Part model, mm, in its own coordinate system. Face numbers are marked on the shaded views. A direction names the side the tool comes from. Round coordinates to 2 decimals unless told otherwise and drop trailing zeros. Order: outer loops, then holes, each group sorted by start corner. A loop starts at its lowest first (then second) coordinate and runs counter-clockwise, first axis right, second up. Notation, with made-up numbers: (28.5, 34.25) -> (58.5, 34.25) arc R33 cw to (58.5, 69.25) -> close; hole circle Ø5 at (23.25, 42.25). An arc over 180 degrees is marked (long way). Use CSV: the item, a comma, the result in double quotes.
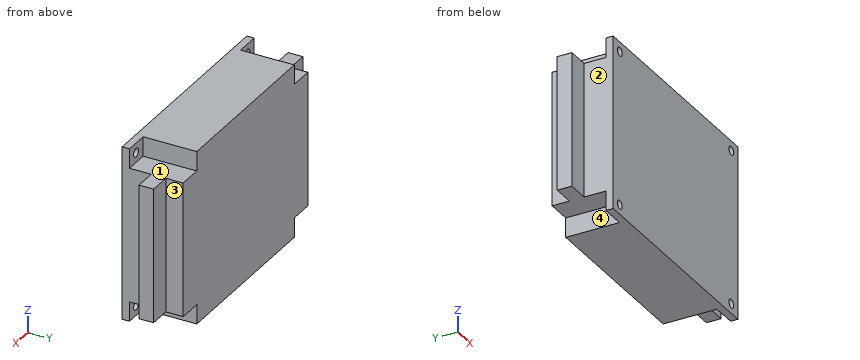
```python
from build123d import *

# Parameters (mm, degrees)
SKETCH_1_W             = 91.7
SKETCH_1_H             = 71
EXTRUDE_1_DEPTH        = 25
SKETCH_2_W             = 10.00292335
SKETCH_2_H             = 22
CUT_EXTRUDE_1_DEPTH    = 8.000270383
SKETCH_3_W             = 54.999459234
SKETCH_3_H             = 13.1
EXTRUDE_2_DEPTH        = 9
SKETCH_4_W             = 8.000270383
SKETCH_4_H             = 22
CUT_EXTRUDE_2_DEPTH    = 10.00292335
SKETCH_5_W             = 8.000270383
SKETCH_5_H             = 22
CUT_EXTRUDE_3_DEPTH    = 10.00292335
SKETCH_6_W             = 54.999459234
SKETCH_6_H             = 13.1
EXTRUDE_3_DEPTH        = 9
SKETCH_7_W             = 8.000270383
SKETCH_7_H             = 22
CUT_EXTRUDE_4_DEPTH    = 10.00292335
SKETCH_8_W             = 9
SKETCH_8_H             = 7.1
CUT_EXTRUDE_5_DEPTH    = 122.38556723
SKETCH_9_W             = 9
SKETCH_9_H             = 7.1
CUT_EXTRUDE_6_DEPTH    = 122.38556723
HOLE_WIZARD_M3_1_D     = 3.531196766
HOLE_WIZARD_M3_1_DEPTH = 25


with BuildPart() as part:
    # 草图1 → 凸台-拉伸1 (new body)
    with BuildSketch(Plane(origin=(0, 25, 0), x_dir=(1, 0, 0), z_dir=(0, 1, 0))):
        with Locations((45.85, 24.5)):
            Rectangle(SKETCH_1_W, SKETCH_1_H)
    extrude(amount=-EXTRUDE_1_DEPTH)

    # 草图2 → 切除-拉伸1 (cut)
    with BuildSketch(Plane(origin=(0, 0, -60), x_dir=(-1, 0, 0), z_dir=(0, 0, -1))):
        with Locations((-5.001461675, 14)):
            Rectangle(SKETCH_2_W, SKETCH_2_H)
    extrude(amount=-CUT_EXTRUDE_1_DEPTH, mode=Mode.SUBTRACT)

    # 草图3 → 凸台-拉伸2 (add)
    with BuildSketch(Plane.ZY):
        with Locations((-24.5, 18.45)):
            Rectangle(SKETCH_3_W, SKETCH_3_H)
    extrude(amount=EXTRUDE_2_DEPTH)

    # 草图4 → 切除-拉伸2 (cut)
    with BuildSketch(Plane.ZY):
        with Locations((6.999864808, 14)):
            Rectangle(SKETCH_4_W, SKETCH_4_H)
    extrude(amount=-CUT_EXTRUDE_2_DEPTH, mode=Mode.SUBTRACT)

    # 草图5 → 切除-拉伸3 (cut)
    with BuildSketch(Plane(origin=(91.7, 0, 0), x_dir=(0, 0, -1), z_dir=(1, 0, 0))):
        with Locations((55.999864809, 14)):
            Rectangle(SKETCH_5_W, SKETCH_5_H)
    extrude(amount=-CUT_EXTRUDE_3_DEPTH, mode=Mode.SUBTRACT)

    # 草图6 → 凸台-拉伸3 (add)
    with BuildSketch(Plane(origin=(91.7, 0, 0), x_dir=(0, 0, -1), z_dir=(1, 0, 0))):
        with Locations((24.5, 18.45)):
            Rectangle(SKETCH_6_W, SKETCH_6_H)
    extrude(amount=EXTRUDE_3_DEPTH)

    # 草图7 → 切除-拉伸4 (cut)
    with BuildSketch(Plane(origin=(91.7, 0, 0), x_dir=(0, 0, -1), z_dir=(1, 0, 0))):
        with Locations((-6.999864808, 14)):
            Rectangle(SKETCH_7_W, SKETCH_7_H)
    extrude(amount=-CUT_EXTRUDE_4_DEPTH, mode=Mode.SUBTRACT)

    # 草图8 → 切除-拉伸5 (cut, through all)
    with BuildSketch(Plane(origin=(0, 0, -51.999729617), x_dir=(-1, 0, 0), z_dir=(0, 0, -1))):
        with Locations((4.5, 21.45)):
            Rectangle(SKETCH_8_W, SKETCH_8_H)
    extrude(amount=-CUT_EXTRUDE_5_DEPTH, mode=Mode.SUBTRACT)

    # 草图9 → 切除-拉伸6 (cut, through all)
    with BuildSketch(Plane.XY.offset(2.999729617)):
        with Locations((96.2, 21.45)):
            Rectangle(SKETCH_9_W, SKETCH_9_H)
    extrude(amount=-CUT_EXTRUDE_6_DEPTH, mode=Mode.SUBTRACT)

    # M3 间隙孔1
    with Locations(Plane(origin=(0, 0, 0), x_dir=(-1, 0, 0), z_dir=(0, -1, 0))):
        with Locations((-86.846324066, 55.999601401), (-86.846324066, -6.999601401), (-4.853675934, -6.999601401), (-4.853675934, 55.999601401)):
            Hole(HOLE_WIZARD_M3_1_D / 2, depth=HOLE_WIZARD_M3_1_DEPTH)


solid = part.part
```
(1) Which spindle directions (+Z, -Z, +X, -X, +Y, -Y) get a long thin tool onto all of the face, cutting with end or side? Do the marked faces 1, 2, 3 and 4. Say none if no direction does.
Reply:
face 1,"+Z, +X, +Y"
face 2,"+Z, -Z, -X, -Y"
face 3,"+Z, -Z, +X, +Y"
face 4,"-Z, -X, +Y"
(2) Probe probe 1 along X at (y, z) = (21, -35.5); probe 2 along X at (y, z) = (14.5, -53.5); probe 3 along Z at (x, y) = (88, 11). List the from-to ranges inside material, lowest first. Write a range as [from, to].
Reply:
probe 1,"[0, 91.7]"
probe 2,"[10, 81.7]"
probe 3,"[-52, 3]"
(3) Cut at A-A, the plane y = 16.25. Give the cut face in (x, z), then the cut area to 3 significant figures.
Reply:
outline,"(-9, -52) -> (10, -52) -> (10, -60) -> (81.7, -60) -> (81.7, -52) -> (100.7, -52) -> (100.7, 3) -> (81.7, 3) -> (81.7, 11) -> (10, 11) -> (10, 3) -> (-9, 3) -> close"
area,"7,180 mm2"
(4) Cut at B-B, the plane z = -11. Give the cut face in (x, y), then the cut area to 3 significant figures.
Reply:
outline,"(-9, 11.9) -> (0, 11.9) -> (0, 0) -> (91.7, 0) -> (91.7, 11.9) -> (100.7, 11.9) -> (100.7, 17.9) -> (91.7, 17.9) -> (91.7, 25) -> (0, 25) -> (0, 17.9) -> (-9, 17.9) -> close"
area,"2,400 mm2"
(5) Drop flat-ended pins along their axis: P1, Ø5.5, axis at x = 3, y = 17, coming from the -Z side; P2, Ø6, axis at y = 5.5, z = -13, coming from the -X side; P3, Ø2.5, axis at x = 4, z = -55.5, coming from the +Y side. Give the stop position or say it passes through.
Reply:
P1,"z = -52"
P2,"x = 0"
P3,"y = 3"
(6) Cut at C-C, the plane x = 87. Give the cut face in (y, z), then the cut area to 3 significant figures.
Reply:
outline,"(0, -60) -> (3, -60) -> (3, -57.76) -> (0, -57.76) -> close; (0, -54.24) -> (3, -54.24) -> (3, -52) -> (25, -52) -> (25, 3) -> (3, 3) -> (3, 5.24) -> (0, 5.24) -> close; (0, 8.76) -> (3, 8.76) -> (3, 11) -> (0, 11) -> close"
area,"1,400 mm2"
